```python
from build123d import *

# Parameters (mm, degrees)
SKETCH2_R          = 5
CUT_EXTRUDE1_DEPTH = 25


with BuildPart() as part:
    # Sketch1 → Revolve1 (revolve)
    with BuildSketch(Plane.XY, mode=Mode.PRIVATE) as revolve1_sk:
        Polygon((67.539059874, 10), (26.539059874, 10), (26.539059874, 16), (39.922105525, 18), (39.922105525, 35), (29.539059874, 38), (29.539059874, 43), (64.539059874, 43), (64.539059874, 38), (54.156014223, 35), (54.156014223, 18), (67.539059874, 16), align=None)
    revolve(revolve1_sk.sketch.rotate(Axis((0, 0, 0), (1, 0, 0)), 90), axis=Axis((0, 0, 0), (1, 0, 0)))

    # Sketch2 → Cut-Extrude1 (cut)
    with BuildSketch(Plane(origin=(54.156014223, 0, 0), x_dir=(0, 0, -1), z_dir=(1, 0, 0))):
        with Locations((0, 26.5)):
            Circle(SKETCH2_R)
        with Locations((26.5, 0)):
            Circle(SKETCH2_R)
        with Locations((0, -26.5)):
            Circle(SKETCH2_R)
        with Locations((-26.5, 0)):
            Circle(SKETCH2_R)
    extrude(amount=-CUT_EXTRUDE1_DEPTH, mode=Mode.SUBTRACT)


solid = part.part
```
Design review of the part built by this model. Coordinates are the model's own, in mm. A direction names the side the tool comes from. Give positions to 0.01 mm unless a question says otherwise; leave off trailing zeros. Write each loop counter-clockwise with the first axis right and the second up, starting at its lowest first coordinate (ties: lowest second). Pieces come first, ordered by that corner, then holes.
(1) Add section B-B (x = 41). Give the boundary of the cut face in (y, z).
Checked values:
outline: circle Ø86 at (0, 0); hole circle Ø10 at (-26.5, 0); hole circle Ø20 at (0, 0); hole circle Ø10 at (0, -26.5); hole circle Ø10 at (0, 26.5); hole circle Ø10 at (26.5, 0)
(2) Clearance check with flat-ended pins moving along their axes: pin 1 Ø1.5 at (x, z) = (57, 34) entering from +Y; pin 2 Ø5 at (x, y) = (34.5, -13) entering from +Z; pin 3 Ø5 at (x, z) = (32.5, -27.5) entering from -Y; pin 4 Ø9 at (y, z) = (26.5, 0) entering from +X. State where each tip first meets the part, or that it passes through.
Checked values:
pin 1: stops at y = 27.27
pin 2: stops at z = 41.7
pin 3: stops at y = -34.99
pin 4: passes through
(3) Add section C-C (x = 58). Give the boundary of the cut face in (y, z), and give its area (3 significant figures).
Checked values:
outline: circle Ø86 at (0, 0); circle Ø34.85 at (0, 0); hole circle Ø72.22 at (0, 0); hole circle Ø20 at (0, 0)
area: 2,350 mm2
(4) Add section D-D (x = 35). Give the boundary of the cut face in (y, z), and give its area (3 significant figures).
Checked values:
outline: circle Ø86 at (0, 0); circle Ø34.53 at (0, 0); hole circle Ø72.84 at (0, 0); hole circle Ø20 at (0, 0)
area: 2,260 mm2
(5) Mouldability with a two-part tool opening along Y and no side actions: class faces 4 (the face through (39.273, -10.569, 33.563)), 5 (the face through (29.539, 35, -16)), 6 (the face through (47.284, -42.634, -5.598)) as +Y half, -Y half, draft (parallel to the pull), parting line (faces both ways), or undercut.
Checked values:
face 4: undercut
face 5: draft
face 6: parting line
(6) Add section A-A (z = 0). Give the number of separate pieces and of enclosed holes in the cut face, and give its area (3 significant figures).
Checked values:
separate pieces: 4
enclosed holes: 0
area: 1,300 mm2
(7) Tool access review of faces 1 (the face through (64.539, 35, 16)), 2 (the face through (39.922, 15, -15)), 3 (the face through (26.539, -0.2, -10.4)): name each direction out of +Z, -Z, +X, -X, +Y, -Y from which nothing blocks a thin tool from reaching the whole face with its end or side.
Checked values:
face 1: +X
face 2: -X
face 3: +Z, -Z, -X, +Y, -Y
(8) Wall thickness on line 1 along Y through (x, z) = (45, 0); line 2 along Y through (x, z) = (38, 0); line 3 along Z through (x, y) = (37.5, -8): over which ranges is each line inside the solid? List them lowest first.
Checked values:
line 1: y = -43 to -31.5, -21.5 to -10, 10 to 21.5, 31.5 to 43
line 2: y = -43 to -35.56, -17.71 to -10, 10 to 17.71, 35.56 to 43
line 3: z = -42.25 to -34.79, -15.72 to -6, 6 to 15.72, 34.79 to 42.25
